Work out the finished part from the listing and answer in its coordinate system (mm). Face numbers are marked on the shaded views. Round coordinates to 2 decimals unless told otherwise and drop trailing zeros. Loops run counter-clockwise (first coordinate to the right, second up) from the corner with the lowest first, then second, coordinate; pieces in that order, holes last.
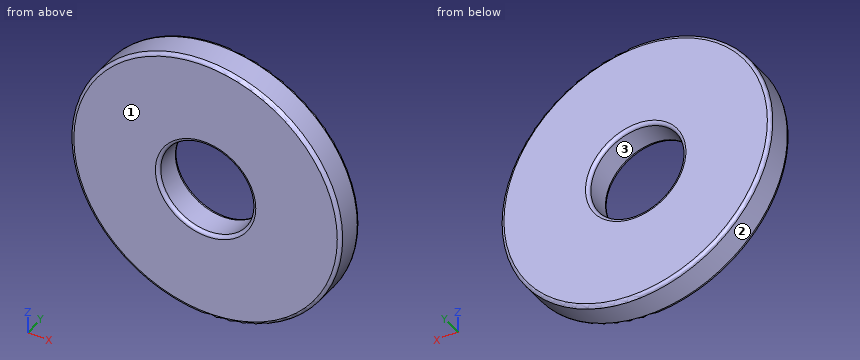
```python
from build123d import *

# Parameters (mm, degrees)
SKETCH1_R           = 5.1562
SKETCH1_R_2         = 1.7907
BOSS_EXTRUDE1_DEPTH = 1.143
FILLET1_R           = 0.127
FILLET2_R           = 0.127
FILLET3_R           = 0.127


with BuildPart() as part:
    # Sketch1 → Boss-Extrude1 (new body)
    with BuildSketch(Plane(origin=(0, 0, 0), x_dir=(1, 0, 0), z_dir=(0, 1, 0))):
        Circle(SKETCH1_R)
        Circle(SKETCH1_R_2, mode=Mode.SUBTRACT)
    extrude(amount=BOSS_EXTRUDE1_DEPTH)

    # Fillet1
    fillet1_edges = [part.edges().sort_by_distance(p)[0] for p in [
        (-5.1562, 1.143, 0),
    ]]
    fillet(fillet1_edges, radius=FILLET1_R)

    # Fillet2
    fillet2_edges = [part.edges().sort_by_distance(p)[0] for p in [
        (-5.1562, 0, 0),
    ]]
    fillet(fillet2_edges, radius=FILLET2_R)

    # Fillet3
    fillet3_edges = [part.edges().sort_by_distance(p)[0] for p in [
        (-1.7907, 0, 0),
        (-1.7907, 1.143, 0),
    ]]
    fillet(fillet3_edges, radius=FILLET3_R)


solid = part.part
```
1. Find section A-A (x = 0). Write down the section's boundary in (y, z).
Answer key:
outline: (0, -5.03) arc R0.13 ccw to (0.13, -5.16) - (1.02, -5.16) arc R0.13 ccw to (1.14, -5.03) - (1.14, -1.92) arc R0.13 ccw to (1.02, -1.79) - (0.13, -1.79) arc R0.13 ccw to (0, -1.92) - close; (0, 1.92) arc R0.13 ccw to (0.13, 1.79) - (1.02, 1.79) arc R0.13 ccw to (1.14, 1.92) - (1.14, 5.03) arc R0.13 ccw to (1.02, 5.16) - (0.13, 5.16) arc R0.13 ccw to (0, 5.03) - close
2. Determine the mould class of the marked faces 1, 2 and 3 for opening direction Z: +Z half, -Z half, draft (parallel to the pull), parting line (faces both ways), or undercut.
Answer key:
face 1: draft
face 2: parting line
face 3: undercut
3. Consider probe 1 along Z at (x, y) = (0, 0.75); probe 2 along Z at (x, y) = (-1, 0.85). Determine where each line is inside the solid, lowest interval first.
Answer key:
probe 1: z = -5.16 to -1.79, 1.79 to 5.16
probe 2: z = -5.06 to -1.49, 1.49 to 5.06
4. Find section B-B (z = 0). Write down the section's boundary in (x, y).
Answer key:
outline: (-5.16, 0.13) arc R0.13 ccw to (-5.03, 0) - (-1.92, 0) arc R0.13 ccw to (-1.79, 0.13) - (-1.79, 1.02) arc R0.13 ccw to (-1.92, 1.14) - (-5.03, 1.14) arc R0.13 ccw to (-5.16, 1.02) - close; (1.79, 0.13) arc R0.13 ccw to (1.92, 0) - (5.03, 0) arc R0.13 ccw to (5.16, 0.13) - (5.16, 1.02) arc R0.13 ccw to (5.03, 1.14) - (1.92, 1.14) arc R0.13 ccw to (1.79, 1.02) - close
5. Find section C-C (y = 0.65). Write down the section's boundary in (x, z).
Answer key:
outline: circle Ø10.31 at (0, 0); hole circle Ø3.58 at (0, 0)
